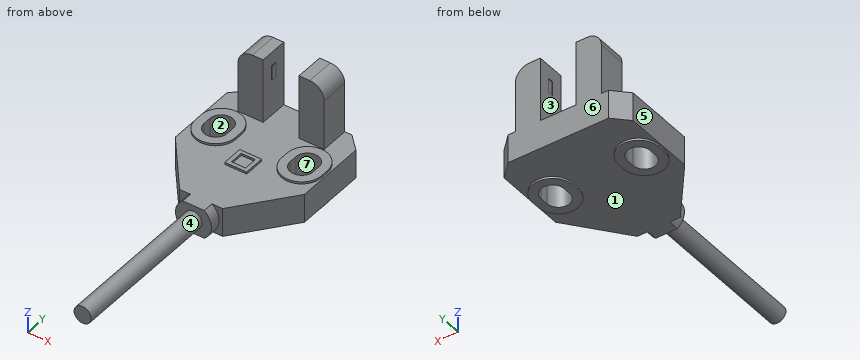
from build123d import *

# Parameters (mm, degrees)
EXTRUDE_1_DEPTH     = 4
EXTRUDE_2_DEPTH     = 4
EXTRUDE_3_DEPTH     = 1.5
SKETCH_4_R          = 1.2
EXTRUDE_4_DEPTH     = 21.5
CHAMFER_1_SIZE      = 2
SKETCH_5_W          = 2
SKETCH_5_H          = 0.8
EXTRUDE_7_DEPTH     = 0.1
SKETCH_6_W          = 2
SKETCH_6_H          = 0.8
CUT_EXTRUDE_2_DEPTH = 0.1
CUT_EXTRUDE_3_REACH = 46.365
EXTRUDE_START       = 0.3
EXTRUDE_8_DEPTH     = 0.3
EXTRUDE_9_DEPTH     = 0.3
SKETCH_10_W         = 3.044276786
SKETCH_10_H         = 2.889483051
SKETCH_10_W_2       = 1.964865926
SKETCH_10_H_2       = 1.90912273
EXTRUDE_10_DEPTH    = 0.3


with BuildPart() as part:
    # 草圖1 → 伸長1 (new body)
    with BuildSketch(Plane.XY):
        Polygon((-9, 0), (9, 0), (9, -12), (3, -19.5), (-3, -19.5), (-9, -12), align=None)
    extrude(amount=EXTRUDE_1_DEPTH)

    # 草圖2 → 伸長2 (add)
    with BuildSketch(Plane(origin=(0, 0, 0), x_dir=(1, 0, 0), z_dir=(0, 1, 0))):
        with BuildLine():
            Line((-6, -4), (-2.5, -4))
            Line((-2.5, -4), (-2.5, -13))
            Line((-2.5, -13), (-4, -13))
            ThreePointArc((-4, -13), (-5.414213562, -12.414213562), (-6, -11))
            Line((-6, -11), (-6, -4))
        make_face()
        with BuildLine():
            Line((2.5, -4), (6, -4))
            Line((6, -4), (6, -11))
            ThreePointArc((6, -11), (5.414213562, -12.414213562), (4, -13))
            Line((4, -13), (2.5, -13))
            Line((2.5, -13), (2.5, -4))
        make_face()
    extrude(amount=-EXTRUDE_2_DEPTH)

    # 草圖3 → 伸長3 (add)
    with BuildSketch(Plane.XZ.offset(19.5)):
        with BuildLine():
            Line((-1.5, 0), (1.5, 0))
            ThreePointArc((1.5, 0), (2.5, 2), (1.5, 4))
            Line((1.5, 4), (-1.5, 4))
            ThreePointArc((-1.5, 4), (-2.5, 2), (-1.5, 0))
        make_face()
    extrude(amount=EXTRUDE_3_DEPTH)

    # 草圖4 → 伸長4 (add)
    with BuildSketch(Plane.XZ.offset(21)):
        with Locations(Location((0, 2, 0), (0, 0, 270))):
            Circle(SKETCH_4_R)
    extrude(amount=EXTRUDE_4_DEPTH)

    # 導角1
    chamfer_1_edges = [part.edges().sort_by_distance(p)[0] for p in [
        (9, 0, 2),
        (-9, 0, 2),
    ]]
    chamfer(chamfer_1_edges, length=CHAMFER_1_SIZE)

    # 草圖5 → 伸長7 (add)
    with BuildSketch(Plane(origin=(-2.5, 0, 0), x_dir=(0, 0, -1), z_dir=(1, 0, 0))):
        with Locations((-10.1, -2)):
            Rectangle(SKETCH_5_W, SKETCH_5_H)
    extrude(amount=EXTRUDE_7_DEPTH)

    # 草圖6 → 除料-伸長2 (cut)
    with BuildSketch(Plane.ZY.offset(-2.5)):
        with Locations((10.1, -2)):
            Rectangle(SKETCH_6_W, SKETCH_6_H)
    extrude(amount=-CUT_EXTRUDE_2_DEPTH, mode=Mode.SUBTRACT)

    # 草圖7 → 除料-伸長3 (cut, up to next)
    with BuildSketch(Plane.XY.offset(4), mode=Mode.PRIVATE) as cut_extrude_3_sk1:
        with BuildLine():
            Line((-7.6, -7.25), (-7.6, -8.35))
            ThreePointArc((-7.6, -8.35), (-6, -9.95), (-4.4, -8.35))
            Line((-4.4, -8.35), (-4.4, -7.25))
            ThreePointArc((-4.4, -7.25), (-6, -5.65), (-7.6, -7.25))
        make_face()
    cut_extrude_3_tool1 = extrude(cut_extrude_3_sk1.sketch, amount=-CUT_EXTRUDE_3_REACH, mode=Mode.PRIVATE) & part.part
    # 草圖7 → 除料-伸長3 (cut, up to next)
    with BuildSketch(Plane.XY.offset(4), mode=Mode.PRIVATE) as cut_extrude_3_sk2:
        with BuildLine():
            Line((4.4, -7.25), (4.4, -8.35))
            ThreePointArc((4.4, -8.35), (6, -9.95), (7.6, -8.35))
            Line((7.6, -8.35), (7.6, -7.25))
            ThreePointArc((7.6, -7.25), (6, -5.65), (4.4, -7.25))
        make_face()
    cut_extrude_3_tool2 = extrude(cut_extrude_3_sk2.sketch, amount=-CUT_EXTRUDE_3_REACH, mode=Mode.PRIVATE) & part.part
    add(cut_extrude_3_tool1.solids().sort_by_distance((-6, -7.8, 4))[0], mode=Mode.SUBTRACT)
    add(cut_extrude_3_tool2.solids().sort_by_distance((6, -7.8, 4))[0], mode=Mode.SUBTRACT)

    # 草圖8 → 伸長8 (add)
    # profile 1 of 2: a face of its own
    with BuildSketch(Plane.XY.offset(4).offset(EXTRUDE_START)):
        with BuildLine():
            Line((3.2, -7.25), (3.2, -8.35))
            ThreePointArc((3.2, -8.35), (6, -11.15), (8.8, -8.35))
            Line((8.8, -8.35), (8.8, -7.25))
            ThreePointArc((8.8, -7.25), (6, -4.45), (3.2, -7.25))
        make_face()
        with BuildLine():
            Line((4.4, -7.25), (4.4, -8.35))
            ThreePointArc((4.4, -8.35), (6, -9.95), (7.6, -8.35))
            Line((7.6, -8.35), (7.6, -7.25))
            ThreePointArc((7.6, -7.25), (6, -5.65), (4.4, -7.25))
        make_face(mode=Mode.SUBTRACT)
    # profile 2 of 2: a face of its own
    with BuildSketch(Plane.XY.offset(4).offset(EXTRUDE_START)):
        with BuildLine():
            Line((-8.8, -7.25), (-8.8, -8.35))
            ThreePointArc((-8.8, -8.35), (-6, -11.15), (-3.2, -8.35))
            Line((-3.2, -8.35), (-3.2, -7.25))
            ThreePointArc((-3.2, -7.25), (-6, -4.45), (-8.8, -7.25))
        make_face()
        with BuildLine():
            Line((-7.6, -7.25), (-7.6, -8.35))
            ThreePointArc((-7.6, -8.35), (-6, -9.95), (-4.4, -8.35))
            Line((-4.4, -8.35), (-4.4, -7.25))
            ThreePointArc((-4.4, -7.25), (-6, -5.65), (-7.6, -7.25))
        make_face(mode=Mode.SUBTRACT)
    extrude(amount=-EXTRUDE_8_DEPTH)

    # 草圖9 → 伸長9 (add)
    # profile 1 of 2: a face of its own
    with BuildSketch(Plane(origin=(0, 0, 0), x_dir=(-1, 0, 0), z_dir=(0, 0, -1))):
        with BuildLine():
            Line((-3.2, -8.35), (-3.2, -7.25))
            ThreePointArc((-3.2, -7.25), (-6, -4.45), (-8.8, -7.25))
            Line((-8.8, -7.25), (-8.8, -8.35))
            ThreePointArc((-8.8, -8.35), (-6, -11.15), (-3.2, -8.35))
        make_face()
        with BuildLine():
            Line((-4.4, -8.35), (-4.4, -7.25))
            ThreePointArc((-4.4, -7.25), (-6, -5.65), (-7.6, -7.25))
            Line((-7.6, -7.25), (-7.6, -8.35))
            ThreePointArc((-7.6, -8.35), (-6, -9.95), (-4.4, -8.35))
        make_face(mode=Mode.SUBTRACT)
    # profile 2 of 2: a face of its own
    with BuildSketch(Plane(origin=(0, 0, 0), x_dir=(-1, 0, 0), z_dir=(0, 0, -1))):
        with BuildLine():
            Line((8.8, -8.35), (8.8, -7.25))
            ThreePointArc((8.8, -7.25), (6, -4.45), (3.2, -7.25))
            Line((3.2, -7.25), (3.2, -8.35))
            ThreePointArc((3.2, -8.35), (6, -11.15), (8.8, -8.35))
        make_face()
        with BuildLine():
            Line((7.6, -8.35), (7.6, -7.25))
            ThreePointArc((7.6, -7.25), (6, -5.65), (4.4, -7.25))
            Line((4.4, -7.25), (4.4, -8.35))
            ThreePointArc((4.4, -8.35), (6, -9.95), (7.6, -8.35))
        make_face(mode=Mode.SUBTRACT)
    extrude(amount=EXTRUDE_9_DEPTH)

    # 草圖10 → 伸長10 (add)
    with BuildSketch(Plane.XY.offset(4)):
        with Locations((-0.011782979, -11.3393837)):
            Rectangle(SKETCH_10_W, SKETCH_10_H)
        with Locations((0, -11.313584744)):
            Rectangle(SKETCH_10_W_2, SKETCH_10_H_2, mode=Mode.SUBTRACT)
    extrude(amount=EXTRUDE_10_DEPTH)


solid = part.part
The listing builds one solid part. Answer for the finished solid, in the listing's coordinates (mm). Face numbers are marked on the shaded views. A direction names the side the tool comes from. Round coordinates to 2 decimals unless told otherwise and drop trailing zeros. Write each loop counter-clockwise with the first axis right and the second up, starting at its lowest first coordinate (ties: lowest second). Pieces come first, ordered by that corner, then holes. Notation, with made-up numbers: M 89.5,-15.75 L 114.5,-15.75 A15 ccw 114.5,1.25 Z; hole C 57,-33 d9. An arc over 180 degrees is marked long. Write each question's results on one line, items separated by ' | '. Start each with the question number.
(1) For the marked faces 1, 2, 3 and 4, determine the directions among +Z, -Z, +X, -X, +Y, -Y from which every point of the face is accessible in a straight line to the end or side of a thin tool.
(2) Find the intervals of material crossed by line 1 (X direction, y = -3, z = 10.5); line 2 (Y direction, x = 7, z = 2.5); line 3 (Z direction, x = -0.75, y = -8), in increasing order.
(3) Each of these flat-tipped pins is pushed along its axis until it touches: P1, Ø1.5, axis at x = 7, z = 10.5, coming from the +Y side; P2, Ø3, axis at x = -7, y = -15.5, coming from the -Z side; P3, Ø4.5, axis at x = 5, y = -8.5, coming from the +Z side; P4, Ø3, axis at y = -1.5, z = 6, coming from the +X side. Where does it stop, or does it pass through?
(4) The part is cut by section C-C, the plane x = 0. Write down the section's boundary in (y, z), and give its area (3 significant figures).
(5) Determine the mould class of the marked faces 5, 6 and 7 for opening direction Y: +Y half, -Y half, draft (parallel to the pull), parting line (faces both ways), or undercut.
(6) The part is cut by section D-D, the plane z = 2. Write down the section's boundary in (x, y), and give its area (3 significant figures).
(7) The part is cut by section A-A, the plane z = 7.5. Write down the section's boundary in (x, y), and give its area (3 significant figures).
(8) The part is cut by section B-B, the plane x = -5. Write down the section's boundary in (y, z), and give its area (3 significant figures).
Worked answers:
1) face 1: -Z | face 2: +Z, -Z | face 3: +Z, +Y, -Y | face 4: -Y
2) line 1: x = -6 to -2.5, 2.5 to 6 | line 2: y = -14.5 to -9.6, -6 to 0 | line 3: z = 0 to 4
3) P1: passes through | P2: stops at z = 0 | P3: stops at z = 4.3 | P4: stops at x = 6
4) outline: M -42.5,0.8 L -21,0.8 L -21,0 L 0,0 L 0,4 L -9.89,4 L -9.89,4.3 L -10.36,4.3 L -10.36,4 L -12.27,4 L -12.27,4.3 L -12.78,4.3 L -12.78,4 L -21,4 L -21,3.2 L -42.5,3.2 Z | area: 136 mm²
5) face 5: draft | face 6: +Y half | face 7: undercut
6) outline: M -9,-12 L -3,-19.5 L -2.5,-19.5 L -2.5,-21 L -1.2,-21 L -1.2,-42.5 L 1.2,-42.5 L 1.2,-21 L 2.5,-21 L 2.5,-19.5 L 3,-19.5 L 9,-12 L 9,-2 L 7,0 L -7,0 L -9,-2 Z; hole M -7.6,-8.35 A1.6 ccw -4.4,-8.35 L -4.4,-7.25 A1.6 ccw -7.6,-7.25 Z; hole M 4.4,-8.35 A1.6 ccw 7.6,-8.35 L 7.6,-7.25 A1.6 ccw 4.4,-7.25 Z | area: 338 mm²
7) outline: M -6,-4 L -2.5,-4 L -2.5,0 L -6,0 Z; M 2.5,-4 L 6,-4 L 6,0 L 2.5,0 Z | area: 28.0 mm²
8) outline: M -17,0 L -10.97,0 L -10.97,-0.3 L -9.6,-0.3 L -9.6,4.3 L -10.97,4.3 L -10.97,4 L -17,4 Z; M -6,-0.3 L -4.63,-0.3 L -4.63,0 L 0,0 L 0,12.73 L -4,12.73 L -4,4 L -4.63,4 L -4.63,4.3 L -6,4.3 Z | area: 90.2 mm²
